```python
from build123d import *

# Parameters (mm, degrees)
BOX001_W      = 4.5
BOX001_H      = 12
BOX001_DEPTH  = 15
ARRAY_X_COUNT = 10
ARRAY_X_PITCH = 15
BOX_W         = 150
BOX_H         = 26
BOX_DEPTH     = 10


with BuildPart() as array:
    # Box001 → Box001 (new body)
    with BuildSketch(Plane(origin=(5, 7, 2), x_dir=(1, 0, 0), z_dir=(0, 0, 1))):
        with Locations((2.25, 6)):
            Rectangle(BOX001_W, BOX001_H)
    extrude(amount=BOX001_DEPTH)

    # Array X: Array ×10


with BuildPart() as array_1:
    add(array.part)
    with Locations(*[(i * ARRAY_X_PITCH, 0, 0) for i in range(1, ARRAY_X_COUNT)]):
        add(array.part)


with BuildPart() as cut:
    # Box → Box (new body)
    with BuildSketch(Plane.XY):
        with Locations((75, 13)):
            Rectangle(BOX_W, BOX_H)
    extrude(amount=BOX_DEPTH)

    # Cut: cut Array
    add(array_1.part, mode=Mode.SUBTRACT)


solid = cut.part
```
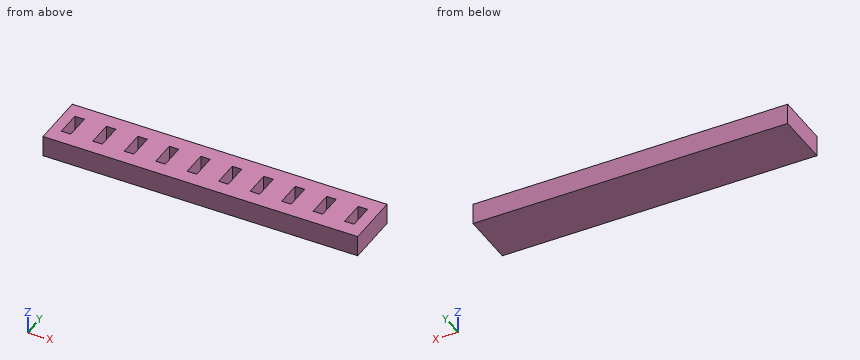
Build history of the part. All positions in model axes, mm. Round coordinates to 2 decimals unless told otherwise and drop trailing zeros. Write each loop counter-clockwise with the first axis right and the second up, starting at its lowest first coordinate (ties: lowest second). Pieces come first, ordered by that corner, then holes.
1) Pin check, flat tips, straight feed: pin 1 (5 mm diameter, centred on y = 16.5, z = 2, fed in from -X); pin 2 (2 mm diameter, centred on x = 66.5, y = 11, fed in from +Z). Stop position of each tip, or through.
2) Band-saw the part on B-B, the plane z = 5.5. Give the number of separate pieces and of enclosed holes in the cut face, and give its area (3 significant figures).
3) Band-saw the part on A-A, the plane x = 141.5. List the corners of the cut face in (y, z), and give its area (3 significant figures).
4) Drill centre lines: probe 1 along Y at (x, z) = (67, 7.25); probe 2 along Z at (x, y) = (8, 14.5). Where is each one in solid material? Low to high.
Ans:
1. pin 1: stops at x = 0
1. pin 2: stops at z = 2
2. separate pieces: 1
2. enclosed holes: 10
2. area: 3,360 mm2
3. outline: (0, 0) - (26, 0) - (26, 10) - (19, 10) - (19, 2) - (7, 2) - (7, 10) - (0, 10) - close
3. area: 164 mm2
4. probe 1: y = 0 to 7, 19 to 26
4. probe 2: z = 0 to 2
